Source: CAD feature listing. Evaluate the final solid. Frame: model axes, mm. A direction names the side the tool comes from. Give positions to 0.01 mm unless a question says otherwise; leave off trailing zeros. Order: outer loops, then holes, each group sorted by start corner. A loop starts at its lowest first (then second) coordinate and runs counter-clockwise, first axis right, second up. Notation, with made-up numbers: M -17,83 L 18,83 A28 cw 18,114 Z; hole C 62,53.5 d7. An arc over 180 degrees is marked long. Use CSV: the item, a comma, the result in double quotes. Start each with the question number.
1. Section query A-A, the plane x = -20.5. Return the cut outline in (y, z), plus the area to 3 significant figures.
2. Pin query (flat end, axial travel): P1, Ø8, axis at x = 12, y = -3, coming from the +Z side; P2, Ø1, axis at y = 5, z = 20.5, coming from the -X side; P3, Ø3, axis at x = 1.5, z = 37.5, coming from the -Y side. Return the tip coordinate at first contact, or that it passes through.
3. Reachability of faces 4 (the cylindrical face through (22.89, 7.21, 27.08)), 5 (the flat face through (-4, 24, 50)) from +Z, -Z, +X, -X, +Y, -Y: full face, straight path, thin tool, end or side. Return the list, or none.
4. Section query B-B, the plane z = 37. Return the cut outline in (x, y), plus the area to 3 significant figures.
5. Line query: line 1 along Y through (x, z) = (0, 15); line 2 along Z through (x, y) = (8, 9); line 3 along Y through (x, z) = (9, 16). Output: solid intervals per line, ascending. Write a range as [from, to].
6. Mould query, pull axis X, two halves, no side actions, for faces 1 (the flat face through (0, -20, 4.8)), 2 (the flat face through (0, 0, -2)), 3 (the flat face through (0, 0, 0)). Classes: released by +X, released by -X, zero draft, split by the parting line, or undercut.
from build123d import *

# Parameters (mm, degrees)
SKETCH1_R           = 26.5
SKETCH1_R_2         = 24
BOSS_EXTRUDE1_DEPTH = 50
BOSS_EXTRUDE2_START = 2
SKETCH2_R           = 26.5
BOSS_EXTRUDE2_DEPTH = 2


with BuildPart() as part:
    # Sketch1 → Boss-Extrude1 (new body)
    with BuildSketch(Plane(origin=(0, 0, 0), x_dir=(0, 1, 0), z_dir=(0, 0, 1))):
        with Locations(Location((0, 0, 0), (0, 0, 270))):
            Circle(SKETCH1_R)
        with Locations(Location((0, 0, 0), (0, 0, 270))):
            Circle(SKETCH1_R_2, mode=Mode.SUBTRACT)
    extrude(amount=BOSS_EXTRUDE1_DEPTH)

    # Sketch2 → Boss-Extrude2 (add)
    with BuildSketch(Plane(origin=(0, 0, 0), x_dir=(1, 0, 0), z_dir=(0, 0, -1)).offset(BOSS_EXTRUDE2_START)):
        with Locations(Location((0, 0, 0), (0, 0, 180))):
            Circle(SKETCH2_R)
    extrude(amount=-BOSS_EXTRUDE2_DEPTH)

    # Sketch5 → Revolve1 (revolve)
    with BuildSketch(Plane.YZ, mode=Mode.PRIVATE) as revolve1_sk:
        with BuildLine():
            Line((-26.5, 0), (-26.5, 4.8))
            Line((-26.5, 4.8), (-19.5, 4.8))
            add(Edge.make_bspline(
                [(-19.5, 4.8), (-19.143895577, 1.941095467), (-17, 0)],
                knots=[0, 0, 0, 1, 1, 1], degree=2))
            Line((-17, 0), (-26.5, 0))
        make_face()
    revolve(revolve1_sk.sketch.rotate(Axis((0, 0, 0), (0, 0, 1)), 270), axis=Axis((0, 0, 0), (0, 0, 1)))


solid = part.part
Result set:
1,outline,"M -16.79,-2 L 16.79,-2 L 16.79,50 L 12.48,50 L 12.48,4.8 L -12.48,4.8 L -12.48,50 L -16.79,50 Z"
1,area,"618 mm2"
2,P1,"z = 0"
2,P2,"x = -26.12"
2,P3,"y = -26.5"
3,face 4,"+Z"
3,face 5,"+Z, +X, -X, +Y, -Y"
4,outline,"C 0,0 d53; hole C 0,0 d48"
4,area,"397 mm2"
5,line 1,"[-26.5, -24], [24, 26.5]"
5,line 2,"[-2, 0]"
5,line 3,"[-24.92, -22.25], [22.25, 24.92]"
6,face 1,"undercut"
6,face 2,"zero draft"
6,face 3,"undercut"
